Verification items for the finished model (mm, model axes). Coordinates: 2 decimals unless noted, no trailing zeros. Loops run counter-clockwise (first coordinate to the right, second up) from the corner with the lowest first, then second, coordinate; pieces in that order, holes last. Notation, with made-up numbers: (3, 57.5) -> (8, 57.5) arc R21 cw to (8, 68.5) -> close; hole circle Ø6 at (-11.75, 28.25). An arc over 180 degrees is marked (long way). Write item = value, one per line.
```python
from build123d import *

# Parameters (mm, degrees)
SKETCH1_W           = 3
SKETCH1_H           = 30
BOSS_EXTRUDE1_DEPTH = 3
SKETCH2_R           = 2
SKETCH2_R_2         = 4
CUT_EXTRUDE1_DEPTH  = 3


with BuildPart() as part:
    # Sketch1 → Boss-Extrude1 (new body)
    with BuildSketch(Plane(origin=(0, 0, 0), x_dir=(1, 0, 0), z_dir=(0, 1, 0))):
        Polygon((-53.189189189, 52.918918919), (-53.189189189, 55.918918919), (-33.189189189, 55.918918919), (-33.189189189, 52.918918919), (-13.189189189, 52.918918919), (-13.189189189, 55.918918919), (6.810810811, 55.918918919), (6.810810811, 52.918918919), (26.810810811, 52.918918919), (26.810810811, 55.918918919), (46.810810811, 55.918918919), (46.810810811, 52.918918919), (66.810810811, 52.918918919), (66.810810811, 55.918918919), (86.810810811, 55.918918919), (86.810810811, 52.918918919), (106.810810811, 52.918918919), (109.810810811, 52.918918919), (109.810810811, 22.918918919), (106.810810811, 22.918918919), (106.810810811, -7.081081081), (109.810810811, -7.081081081), (109.810810811, -37.081081081), (106.810810811, -37.081081081), (106.810810811, -40.081081081), (86.810810811, -40.081081081), (86.810810811, -37.081081081), (66.810810811, -37.081081081), (66.810810811, -40.081081081), (46.810810811, -40.081081081), (46.810810811, -37.081081081), (26.810810811, -37.081081081), (26.810810811, -40.081081081), (6.810810811, -40.081081081), (6.810810811, -37.081081081), (-13.189189189, -37.081081081), (-13.189189189, -40.081081081), (-33.189189189, -40.081081081), (-33.189189189, -37.081081081), (-53.189189189, -37.081081081), (-53.189189189, -40.081081081), (-73.189189189, -40.081081081), (-73.189189189, -37.081081081), (-93.189189189, -37.081081081), (-96.189189189, -37.081081081), (-96.189189189, -7.081081081), (-93.189189189, -7.081081081), (-93.189189189, 22.918918919), (-96.189189189, 22.918918919), (-96.189189189, 52.918918919), (-93.189189189, 52.918918919), (-93.189189189, 55.918918919), (-73.189189189, 55.918918919), (-73.189189189, 52.918918919), align=None)
        with Locations((6.810810811, 7.918918919)):
            Rectangle(SKETCH1_W, SKETCH1_H, mode=Mode.SUBTRACT)
    extrude(amount=BOSS_EXTRUDE1_DEPTH)

    # Sketch2 → Cut-Extrude1 (cut)
    with BuildSketch(Plane(origin=(0, 3, 0), x_dir=(1, 0, 0), z_dir=(0, 1, 0))):
        with Locations(Location((-83.189189189, 47.918918919, 0), (0, 0, 270))):
            Circle(SKETCH2_R)
        with Locations(Location((-83.189189189, -32.081081081, 0), (0, 0, 270))):
            Circle(SKETCH2_R)
        with Locations(Location((-3.189189189, 47.918918919, 0), (0, 0, 270))):
            Circle(SKETCH2_R)
        with Locations(Location((-3.189189189, -32.081081081, 0), (0, 0, 270))):
            Circle(SKETCH2_R)
        with Locations(Location((96.97523931, 47.753811706, 0), (0, 0, 270))):
            Circle(SKETCH2_R)
        with Locations(Location((96.890661701, -31.999841307, 0), (0, 0, 270))):
            Circle(SKETCH2_R)
        with Locations(Location((16.73095992, 47.837679145, 0), (0, 0, 270))):
            Circle(SKETCH2_R)
        with Locations(Location((16.92956487, -32.199971625, 0), (0, 0, 270))):
            Circle(SKETCH2_R)
        with Locations(Location((64.409536285, 15.225493569, 0), (0, 0, 270))):
            Circle(SKETCH2_R_2)
        with Locations(Location((64.458960542, 0.301508961, 0), (0, 0, 270))):
            Circle(SKETCH2_R_2)
        with Locations(Location((72.150575188, 22.957645887, 0), (0, 0, 270))):
            Circle(SKETCH2_R_2)
        with Locations(Location((79.984903702, 30.782980722, 0), (0, 0, 270))):
            Circle(SKETCH2_R_2)
        with Locations(Location((42.782150533, -6.377064303, 0), (0, 0, 270))):
            Circle(SKETCH2_R_2)
        with Locations(Location((35.744744462, -13.406391548, 0), (0, 0, 270))):
            Circle(SKETCH2_R_2)
        with Locations(Location((50.031602385, 0.251885254, 0), (0, 0, 270))):
            Circle(SKETCH2_R_2)
        with Locations(Location((71.328743505, -6.540662674, 0), (0, 0, 270))):
            Circle(SKETCH2_R_2)
        with Locations(Location((56.810810811, 7.918918919, 0), (0, 0, 270))):
            Circle(SKETCH2_R_2)
        with Locations(Location((79.984903702, -15.162031659, 0), (0, 0, 270))):
            Circle(SKETCH2_R_2)
        with Locations(Location((50.031602385, 14.670880058, 0), (0, 0, 270))):
            Circle(SKETCH2_R_2)
        with Locations(Location((42.782150533, 21.891194601, 0), (0, 0, 270))):
            Circle(SKETCH2_R_2)
        with Locations(Location((33.854481941, 30.782980722, 0), (0, 0, 270))):
            Circle(SKETCH2_R_2)
        with Locations(Location((70.286929504, 7.918918919, 0), (0, 0, 270))):
            Circle(SKETCH2_R_2)
        with Locations(Location((80.695917052, 7.918918919, 0), (0, 0, 270))):
            Circle(SKETCH2_R_2)
        with Locations(Location((89.69828466, 7.918918919, 0), (0, 0, 270))):
            Circle(SKETCH2_R_2)
        with Locations(Location((35.027656371, 7.918918919, 0), (0, 0, 270))):
            Circle(SKETCH2_R_2)
        with Locations(Location((44.40512263, 7.918918919, 0), (0, 0, 270))):
            Circle(SKETCH2_R_2)
        with Locations(Location((25.368866125, 7.918918919, 0), (0, 0, 270))):
            Circle(SKETCH2_R_2)
        with Locations(Location((57.533575392, -5.280819839, 0), (0, 0, 270))):
            Circle(SKETCH2_R_2)
        with Locations(Location((57.533575392, -15.162031659, 0), (0, 0, 270))):
            Circle(SKETCH2_R_2)
        with Locations(Location((57.533575392, -24.410851007, 0), (0, 0, 270))):
            Circle(SKETCH2_R_2)
        with Locations(Location((56.810810811, 21.891194601, 0), (0, 0, 270))):
            Circle(SKETCH2_R_2)
        with Locations(Location((56.810810811, 31.666397221, 0), (0, 0, 270))):
            Circle(SKETCH2_R_2)
        with Locations(Location((56.810810811, 40.762539492, 0), (0, 0, 270))):
            Circle(SKETCH2_R_2)
        with Locations(Location((33.854481941, 18.444169796, 0), (0, 0, 270))):
            Circle(SKETCH2_R_2)
        with Locations(Location((46.782150533, 34.292087773, 0), (0, 0, 270))):
            Circle(SKETCH2_R_2)
        with Locations(Location((68.786534903, 34.292087773, 0), (0, 0, 270))):
            Circle(SKETCH2_R_2)
        with Locations(Location((82.102536991, 18.670880058, 0), (0, 0, 270))):
            Circle(SKETCH2_R_2)
        with Locations(Location((81.446114352, -3.030227937, 0), (0, 0, 270))):
            Circle(SKETCH2_R_2)
        with Locations(Location((67.661238952, -17.096427325, 0), (0, 0, 270))):
            Circle(SKETCH2_R_2)
        with Locations(Location((46.782150533, -17.096427325, 0), (0, 0, 270))):
            Circle(SKETCH2_R_2)
        with Locations(Location((33.854481941, -3.030227937, 0), (0, 0, 270))):
            Circle(SKETCH2_R_2)
        with Locations(Location((-35.761406417, 15.18771879, 0), (0, 0, 270))):
            Circle(SKETCH2_R_2)
        with Locations(Location((-35.71198216, 0.263734182, 0), (0, 0, 270))):
            Circle(SKETCH2_R_2)
        with Locations(Location((-28.020367515, 22.919871108, 0), (0, 0, 270))):
            Circle(SKETCH2_R_2)
        with Locations(Location((-20.186039001, 30.745205943, 0), (0, 0, 270))):
            Circle(SKETCH2_R_2)
        with Locations(Location((-57.388792169, -6.414839082, 0), (0, 0, 270))):
            Circle(SKETCH2_R_2)
        with Locations(Location((-64.42619824, -13.444166327, 0), (0, 0, 270))):
            Circle(SKETCH2_R_2)
        with Locations(Location((-50.139340317, 0.214110475, 0), (0, 0, 270))):
            Circle(SKETCH2_R_2)
        with Locations(Location((-28.842199198, -6.578437453, 0), (0, 0, 270))):
            Circle(SKETCH2_R_2)
        with Locations(Location((-43.360131891, 7.88114414, 0), (0, 0, 270))):
            Circle(SKETCH2_R_2)
        with Locations(Location((-20.186039001, -15.199806438, 0), (0, 0, 270))):
            Circle(SKETCH2_R_2)
        with Locations(Location((-50.139340317, 14.633105278, 0), (0, 0, 270))):
            Circle(SKETCH2_R_2)
        with Locations(Location((-57.388792169, 21.853419822, 0), (0, 0, 270))):
            Circle(SKETCH2_R_2)
        with Locations(Location((-66.316460761, 30.745205943, 0), (0, 0, 270))):
            Circle(SKETCH2_R_2)
        with Locations(Location((-29.884013198, 7.88114414, 0), (0, 0, 270))):
            Circle(SKETCH2_R_2)
        with Locations(Location((-19.475025651, 7.88114414, 0), (0, 0, 270))):
            Circle(SKETCH2_R_2)
        with Locations(Location((-10.472658042, 7.88114414, 0), (0, 0, 270))):
            Circle(SKETCH2_R_2)
        with Locations(Location((-65.143286331, 7.88114414, 0), (0, 0, 270))):
            Circle(SKETCH2_R_2)
        with Locations(Location((-55.765820072, 7.88114414, 0), (0, 0, 270))):
            Circle(SKETCH2_R_2)
        with Locations(Location((-74.802076578, 7.88114414, 0), (0, 0, 270))):
            Circle(SKETCH2_R_2)
        with Locations(Location((-42.63736731, -5.318594618, 0), (0, 0, 270))):
            Circle(SKETCH2_R_2)
        with Locations(Location((-42.63736731, -15.199806438, 0), (0, 0, 270))):
            Circle(SKETCH2_R_2)
        with Locations(Location((-42.63736731, -24.448625786, 0), (0, 0, 270))):
            Circle(SKETCH2_R_2)
        with Locations(Location((-43.360131891, 21.853419822, 0), (0, 0, 270))):
            Circle(SKETCH2_R_2)
        with Locations(Location((-43.360131891, 31.628622442, 0), (0, 0, 270))):
            Circle(SKETCH2_R_2)
        with Locations(Location((-43.360131891, 40.724764713, 0), (0, 0, 270))):
            Circle(SKETCH2_R_2)
        with Locations(Location((-66.316460761, 18.406395017, 0), (0, 0, 270))):
            Circle(SKETCH2_R_2)
        with Locations(Location((-53.388792169, 34.254312994, 0), (0, 0, 270))):
            Circle(SKETCH2_R_2)
        with Locations(Location((-31.384407799, 34.254312994, 0), (0, 0, 270))):
            Circle(SKETCH2_R_2)
        with Locations(Location((-18.068405712, 18.633105278, 0), (0, 0, 270))):
            Circle(SKETCH2_R_2)
        with Locations(Location((-18.72482835, -3.068002716, 0), (0, 0, 270))):
            Circle(SKETCH2_R_2)
        with Locations(Location((-32.50970375, -17.134202104, 0), (0, 0, 270))):
            Circle(SKETCH2_R_2)
        with Locations(Location((-53.388792169, -17.134202104, 0), (0, 0, 270))):
            Circle(SKETCH2_R_2)
        with Locations(Location((-66.316460761, -3.068002716, 0), (0, 0, 270))):
            Circle(SKETCH2_R_2)
    extrude(amount=-CUT_EXTRUDE1_DEPTH, mode=Mode.SUBTRACT)


solid = part.part
```
1) Sectioned sample at B-B, the plane z = 15. Count the separate pieces of the cut face and the enclosed holes in it, plus the area to 4 significant figures.
Ans:
separate_pieces = 11
enclosed_holes = 0
area = 396.5 mm2
2) Material ranges on line 1 (X direction, y = 1.2, z = 33); line 2 (X direction, y = 2.85, z = 25.5); line 3 (Z direction, x = 47, y = 2.1), recorded low to high.
Ans:
line_1 = -96.19 to -84.97, -81.41 to -4.97, -1.41 to 15.1, 18.76 to 95.16, 98.62 to 109.81
line_2 = -96.19 to -46.5, -38.78 to 53.68, 61.38 to 109.81
line_3 = -52.92 to -38.29, -30.3 to -17.28, -12.06 to -10.96, -4.87 to -2.86, 2.36 to 13.1, 21.09 to 40.08
3) Sectioned sample at A-A, the plane z = 25.5. Record the cut outline in (x, y), plus the area to 3 significant figures.
Ans:
outline = (-96.19, 0) -> (-46.5, 0) -> (-46.5, 3) -> (-96.19, 3) -> close; (-38.78, 0) -> (53.68, 0) -> (53.68, 3) -> (-38.78, 3) -> close; (61.38, 0) -> (109.81, 0) -> (109.81, 3) -> (61.38, 3) -> close
area = 572 mm2
